Verification items for the finished model (mm, model axes). A direction names the side the tool comes from. Coordinates: 2 decimals unless noted, no trailing zeros. Order: outer loops, then holes, each group sorted by start corner. A loop starts at its lowest first (then second) coordinate and runs counter-clockwise, first axis right, second up. Notation, with made-up numbers: (68.25, -3) -> (116.25, -3) arc R19 cw to (116.25, 8) -> close; hole circle Ø2 at (-19.75, -12). An arc over 180 degrees is marked (long way). Answer as CSV lines item,"result".
```python
from build123d import *

# Parameters (mm, degrees)
SKETCH1_R           = 7
SKETCH1_R_2         = 5.5
BOSS_EXTRUDE1_DEPTH = 2.5
SKETCH2_R           = 1
BOSS_EXTRUDE2_DEPTH = 0.75
FILLET1_R           = 1


with BuildPart() as part:
    # Sketch1 → Boss-Extrude1 (new, symmetric)
    with BuildSketch(Plane(origin=(0, 0, 0), x_dir=(1, 0, 0), z_dir=(0, 1, 0))):
        with Locations(Location((0, 0, 0), (0, 0, 270))):
            Circle(SKETCH1_R)
        with Locations(Location((0, 0, 0), (0, 0, 270))):
            Circle(SKETCH1_R_2, mode=Mode.SUBTRACT)
    extrude(amount=BOSS_EXTRUDE1_DEPTH, both=True)

    # Sketch2 → Boss-Extrude2 (add, symmetric)
    with BuildSketch(Plane(origin=(0, 0, 0), x_dir=(1, 0, 0), z_dir=(0, 1, 0))):
        with BuildLine():
            Line((2.595653006, -40), (2.595653006, -6.500968041))
            ThreePointArc((2.595653006, -6.500968041), (0.102408357, -6.999250855), (-2.404346994, -6.574124697))
            Line((-2.404346994, -6.574124697), (-2.404346994, -40))
            ThreePointArc((-2.404346994, -40), (0.095653006, -42.5), (2.595653006, -40))
        make_face()
        with Locations(Location((0.095653006, -40, 0), (0, 0, 270))):
            Circle(SKETCH2_R, mode=Mode.SUBTRACT)
    extrude(amount=BOSS_EXTRUDE2_DEPTH, both=True)

    # Fillet1
    fillet1_edges = [part.edges().sort_by_distance(p)[0] for p in [
        (1.321594437, 0.75, 6.874109989),
        (1.321594437, -0.75, 6.874109989),
    ]]
    fillet(fillet1_edges, radius=FILLET1_R)


solid = part.part
```
Item 1: Tool access check on faces 4 (the flat face through (2.596, 0, 23)), 5 (the cylindrical face through (0.396, -0.01, 40.954)), 6 (the flat face through (0, -0.75, 25)), 7 (the flat face through (-2.404, 0, 23)), 8 (the flat face through (0, 0.75, 25)). Record the directions out of +Z, -Z, +X, -X, +Y, -Y that give a thin tool (end or side, any length) a straight path to the whole face; none if there is none.
Answer list:
face 4,"+Z, +X, +Y, -Y"
face 5,"+Y, -Y"
face 6,"+Z, +X, -X, -Y"
face 7,"+Z, -X, +Y, -Y"
face 8,"+Z, +X, -X, +Y"
Item 2: Thickness scan on line 1 (X direction, y = 0.3, z = 40); line 2 (X direction, y = -0.9, z = 0); line 3 (Z direction, x = 0.75, y = 0.55). Record the ranges inside material, lowest first.
Answer list:
line 1,"-2.4 to -0.9, 1.1 to 2.6"
line 2,"-7 to -5.5, 5.5 to 7"
line 3,"-6.96 to -5.45, 5.45 to 39.24, 40.76 to 42.41"
Item 3: Section check D-D, the plane z = 28. Record the boundary of the cut face in (x, y).
Answer list:
outline,"(-2.4, -0.75) -> (2.6, -0.75) -> (2.6, 0.75) -> (-2.4, 0.75) -> close"
Item 4: Section check A-A, the plane z = 0. Record the boundary of the cut face in (x, y), plus the area to 3 significant figures.
Answer list:
outline,"(-7, -2.5) -> (-5.5, -2.5) -> (-5.5, 2.5) -> (-7, 2.5) -> close; (5.5, -2.5) -> (7, -2.5) -> (7, 2.5) -> (5.5, 2.5) -> close"
area,"15.0 mm2"
Item 5: Section check B-B, the plane x = -4.5. Record the boundary of the cut face in (y, z), plus the area to 3 significant figures.
Answer list:
outline,"(-2.5, -5.36) -> (2.5, -5.36) -> (2.5, -3.16) -> (-2.5, -3.16) -> close; (-2.5, 3.16) -> (2.5, 3.16) -> (2.5, 5.36) -> (-2.5, 5.36) -> close"
area,"22.0 mm2"
Item 6: Section check C-C, the plane y = 0.1. Record the boundary of the cut face in (x, z), plus the area to 3 significant figures.
Answer list:
outline,"(-2.4, 6.57) arc R7 ccw (long way) to (2.6, 6.5) -> (2.6, 40) arc R2.5 ccw to (-2.4, 40) -> close; hole circle Ø11 at (0, 0); hole circle Ø2 at (0.1, 40)"
area,"231 mm2"
Item 7: Release check for a two-part mould opening along Z. For faces 1 (the cylindrical face through (-5.37, -0.04, -1.19)), 2 (the cylindrical face through (-4.259, 0.035, -5.555)), 3 (the flat face through (-4, -2.5, -4)) record: +Z half, -Z half, draft (parallel to the pull), parting line (faces both ways), or undercut.
Answer list:
face 1,"undercut"
face 2,"parting line"
face 3,"draft"
Item 8: Depth check by flat-ended pin: pin 1 Ø4 at (x, z) = (1.5, 25.5) entering from +Y; pin 2 Ø1.1 at (y, z) = (-1, 25) entering from -X; pin 3 Ø1.8 at (y, z) = (0, 16) entering from +X; pin 4 Ø1 at (x, z) = (4.5, 31.5) entering from -Y (3 decimals). Enter the tip coordinate at first touch or a pass-through.
Answer list:
pin 1,"y = 0.75"
pin 2,"x = -2.4"
pin 3,"x = 2.6"
pin 4,"through"
